```python
from build123d import *

# Parameters (mm, degrees)
EXTRUDE_1_DEPTH     = 3
CUT_EXTRUDE_1_REACH = 67.393
SKETCH_2_R          = 0.75
CUT_EXTRUDE_3_REACH = 67.393
SKETCH_4_W          = 20
SKETCH_4_H          = 6
CUT_EXTRUDE_4_REACH = 67.393
SKETCH_5_W          = 6
SKETCH_5_H          = 20
SKETCH_7_W          = 21
SKETCH_7_H          = 2
CUT_EXTRUDE_6_DEPTH = 13
SKETCH_8_W          = 2
SKETCH_8_H          = 21
CUT_EXTRUDE_7_DEPTH = 13
SKETCH_9_W          = 1.5
SKETCH_9_H          = 25
EXTRUDE_2_DEPTH     = 33


with BuildPart() as part:
    # 草图1 → 凸台-拉伸1 (new body)
    with BuildSketch(Plane.XY):
        Polygon((0, 0), (57.5, 0), (57.5, -29), (29, -29), (29, -31), (0, -31), align=None)
    extrude(amount=EXTRUDE_1_DEPTH)

    # 草图2 → 切除-拉伸1 (cut, up to next)
    with BuildSketch(Plane.XY.offset(3), mode=Mode.PRIVATE) as cut_extrude_1_sk1:
        with Locations((31.05, -4.25)):
            Circle(SKETCH_2_R)
    cut_extrude_1_tool1 = extrude(cut_extrude_1_sk1.sketch, amount=-CUT_EXTRUDE_1_REACH, mode=Mode.PRIVATE) & part.part
    # 草图2 → 切除-拉伸1 (cut, up to next)
    with BuildSketch(Plane.XY.offset(3), mode=Mode.PRIVATE) as cut_extrude_1_sk2:
        with Locations((55.5, -4.25)):
            Circle(SKETCH_2_R)
    cut_extrude_1_tool2 = extrude(cut_extrude_1_sk2.sketch, amount=-CUT_EXTRUDE_1_REACH, mode=Mode.PRIVATE) & part.part
    # 草图2 → 切除-拉伸1 (cut, up to next)
    with BuildSketch(Plane.XY.offset(3), mode=Mode.PRIVATE) as cut_extrude_1_sk3:
        with Locations((31.05, -24.75)):
            Circle(SKETCH_2_R)
    cut_extrude_1_tool3 = extrude(cut_extrude_1_sk3.sketch, amount=-CUT_EXTRUDE_1_REACH, mode=Mode.PRIVATE) & part.part
    # 草图2 → 切除-拉伸1 (cut, up to next)
    with BuildSketch(Plane.XY.offset(3), mode=Mode.PRIVATE) as cut_extrude_1_sk4:
        with Locations((55.5, -24.75)):
            Circle(SKETCH_2_R)
    cut_extrude_1_tool4 = extrude(cut_extrude_1_sk4.sketch, amount=-CUT_EXTRUDE_1_REACH, mode=Mode.PRIVATE) & part.part
    # 草图2 → 切除-拉伸1 (cut, up to next)
    with BuildSketch(Plane.XY.offset(3), mode=Mode.PRIVATE) as cut_extrude_1_sk5:
        with Locations((4.25, -29)):
            Circle(SKETCH_2_R)
    cut_extrude_1_tool5 = extrude(cut_extrude_1_sk5.sketch, amount=-CUT_EXTRUDE_1_REACH, mode=Mode.PRIVATE) & part.part
    # 草图2 → 切除-拉伸1 (cut, up to next)
    with BuildSketch(Plane.XY.offset(3), mode=Mode.PRIVATE) as cut_extrude_1_sk6:
        with Locations((24.75, -29)):
            Circle(SKETCH_2_R)
    cut_extrude_1_tool6 = extrude(cut_extrude_1_sk6.sketch, amount=-CUT_EXTRUDE_1_REACH, mode=Mode.PRIVATE) & part.part
    # 草图2 → 切除-拉伸1 (cut, up to next)
    with BuildSketch(Plane.XY.offset(3), mode=Mode.PRIVATE) as cut_extrude_1_sk7:
        with Locations((4.25, -4.55)):
            Circle(SKETCH_2_R)
    cut_extrude_1_tool7 = extrude(cut_extrude_1_sk7.sketch, amount=-CUT_EXTRUDE_1_REACH, mode=Mode.PRIVATE) & part.part
    # 草图2 → 切除-拉伸1 (cut, up to next)
    with BuildSketch(Plane.XY.offset(3), mode=Mode.PRIVATE) as cut_extrude_1_sk8:
        with Locations((24.75, -4.55)):
            Circle(SKETCH_2_R)
    cut_extrude_1_tool8 = extrude(cut_extrude_1_sk8.sketch, amount=-CUT_EXTRUDE_1_REACH, mode=Mode.PRIVATE) & part.part
    add(cut_extrude_1_tool1.solids().sort_by_distance((31.05, -4.25, 3))[0], mode=Mode.SUBTRACT)
    add(cut_extrude_1_tool2.solids().sort_by_distance((55.5, -4.25, 3))[0], mode=Mode.SUBTRACT)
    add(cut_extrude_1_tool3.solids().sort_by_distance((31.05, -24.75, 3))[0], mode=Mode.SUBTRACT)
    add(cut_extrude_1_tool4.solids().sort_by_distance((55.5, -24.75, 3))[0], mode=Mode.SUBTRACT)
    add(cut_extrude_1_tool5.solids().sort_by_distance((4.25, -29, 3))[0], mode=Mode.SUBTRACT)
    add(cut_extrude_1_tool6.solids().sort_by_distance((24.75, -29, 3))[0], mode=Mode.SUBTRACT)
    add(cut_extrude_1_tool7.solids().sort_by_distance((4.25, -4.55, 3))[0], mode=Mode.SUBTRACT)
    add(cut_extrude_1_tool8.solids().sort_by_distance((24.75, -4.55, 3))[0], mode=Mode.SUBTRACT)

    # 草图4 → 切除-拉伸3 (cut, up to next)
    with BuildSketch(Plane(origin=(0, 0, 0), x_dir=(-1, 0, 0), z_dir=(0, 0, -1)), mode=Mode.PRIVATE) as cut_extrude_3_sk1:
        with Locations((-14.5, -23)):
            Rectangle(SKETCH_4_W, SKETCH_4_H)
    cut_extrude_3_tool1 = extrude(cut_extrude_3_sk1.sketch, amount=-CUT_EXTRUDE_3_REACH, mode=Mode.PRIVATE) & part.part
    add(cut_extrude_3_tool1.solids().sort_by_distance((14.5, -23, 0))[0], mode=Mode.SUBTRACT)

    # 草图5 → 切除-拉伸4 (cut, up to next)
    with BuildSketch(Plane(origin=(0, 0, 0), x_dir=(-1, 0, 0), z_dir=(0, 0, -1)), mode=Mode.PRIVATE) as cut_extrude_4_sk1:
        with Locations((-49.5, -14.5)):
            Rectangle(SKETCH_5_W, SKETCH_5_H)
    cut_extrude_4_tool1 = extrude(cut_extrude_4_sk1.sketch, amount=-CUT_EXTRUDE_4_REACH, mode=Mode.PRIVATE) & part.part
    add(cut_extrude_4_tool1.solids().sort_by_distance((49.5, -14.5, 0))[0], mode=Mode.SUBTRACT)

    # 草图7 → 切除-拉伸6 (cut)
    with BuildSketch(Plane.XZ.offset(20)):
        with Locations((14.5, 2)):
            Rectangle(SKETCH_7_W, SKETCH_7_H)
    extrude(amount=-CUT_EXTRUDE_6_DEPTH, mode=Mode.SUBTRACT)

    # 草图8 → 切除-拉伸7 (cut)
    with BuildSketch(Plane(origin=(46.5, 0, 0), x_dir=(0, 0, -1), z_dir=(1, 0, 0))):
        with Locations((-2, -14.5)):
            Rectangle(SKETCH_8_W, SKETCH_8_H)
    extrude(amount=-CUT_EXTRUDE_7_DEPTH, mode=Mode.SUBTRACT)

    # 草图9 → 凸台-拉伸2 (add)
    with BuildSketch(Plane.XY.offset(3)):
        Polygon((0, -31), (2, -31), (2, -2), (27, -2), (28.5, -2), (57.5, -2), (57.5, 0), (0, 0), align=None)
        with Locations((27.75, -14.5)):
            Rectangle(SKETCH_9_W, SKETCH_9_H)
        Polygon((27, -27), (27, -31), (29, -31), (29, -29), (57.5, -29), (57.5, -27), (28.5, -27), align=None)
    extrude(amount=EXTRUDE_2_DEPTH)


solid = part.part
```
Source: CAD feature listing. Evaluate the final solid. Frame: model axes, mm. A direction names the side the tool comes from. Give positions to 0.01 mm unless a question says otherwise; leave off trailing zeros. Loops run counter-clockwise (first coordinate to the right, second up) from the corner with the lowest first, then second, coordinate; pieces in that order, holes last. Notation, with made-up numbers: (-6, 8.25) -> (17, 8.25) arc R23 ccw to (17, 16.25) -> close; hole circle Ø5 at (14, 16). An arc over 180 degrees is marked (long way). Put each result on its own line as item: value. Start each with the question number.
1) Reachability of faces 1 (the face through (4.5, -23, 1)), 2 (the face through (43, -27, 19)), 3 (the face through (2, -17, 19)) from +Z, -Z, +X, -X, +Y, -Y: full face, straight path, thin tool, end or side. Return the list, or none.
2) Cut plane A-A (y = -22). Return loops of the section in (x, z), then the cut area to 3 significant figures.
3) Cut plane B-B (x = 55.5). Return loops of the section in (y, z).
4) Contact query for flat-ended pins moving along their axis: P1, Ø2, axis at x = 4.25, y = -29, coming from the +Z side; P2, Ø1.6, axis at x = 42.5, z = 2.5, coming from the -Y side; P3, Ø12, axis at y = -18.5, z = 12, coming from the +X side. Output: stop coordinate, or through.
5) Material intervals for probe 1 along Y at (x, z) = (31.05, 2.4); probe 2 along X at (y, z) = (-5, 16.5); probe 3 along X at (y, z) = (-29.5, 23), sorted ascending.
6) Cut plane D-D (x = 6). Return loops of the section in (y, z), then the cut area to 3 significant figures.
7) Cut plane C-C (z = 22.5). Return loops of the section in (x, y).
Results are:
1. face 1: +Z, -Z
1. face 2: +Z, +X
1. face 3: +Z, -Y
2. outline: (0, 0) -> (4.5, 0) -> (4.5, 3) -> (2, 3) -> (2, 36) -> (0, 36) -> close; (24.5, 0) -> (46.5, 0) -> (46.5, 1) -> (33.5, 1) -> (33.5, 3) -> (28.5, 3) -> (28.5, 36) -> (27, 36) -> (27, 3) -> (24.5, 3) -> close; (52.5, 0) -> (57.5, 0) -> (57.5, 3) -> (52.5, 3) -> close
2. area: 184 mm2
3. outline: (-29, 0) -> (-25.5, 0) -> (-25.5, 3) -> (-27, 3) -> (-27, 36) -> (-29, 36) -> close; (-24, 0) -> (-5, 0) -> (-5, 3) -> (-24, 3) -> close; (-3.5, 0) -> (0, 0) -> (0, 36) -> (-2, 36) -> (-2, 3) -> (-3.5, 3) -> close
4. P1: stops at z = 3
4. P2: stops at y = -29
4. P3: stops at x = 28.5
5. probe 1: y = -29 to -25.5, -24 to -5, -3.5 to 0
5. probe 2: x = 0 to 2, 27 to 28.5
5. probe 3: x = 0 to 2, 27 to 29
6. outline: (-31, 0) -> (-26, 0) -> (-26, 3) -> (-31, 3) -> close; (-20, 0) -> (0, 0) -> (0, 36) -> (-2, 36) -> (-2, 3) -> (-7, 3) -> (-7, 1) -> (-20, 1) -> close
6. area: 115 mm2
7. outline: (0, -31) -> (2, -31) -> (2, -2) -> (27, -2) -> (27, -31) -> (29, -31) -> (29, -29) -> (57.5, -29) -> (57.5, -27) -> (28.5, -27) -> (28.5, -2) -> (57.5, -2) -> (57.5, 0) -> (0, 0) -> close
